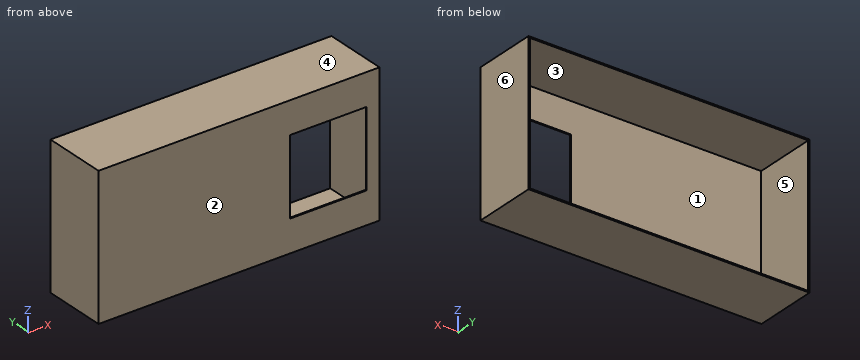
```python
from build123d import *

# Parameters (mm, degrees)
SKETCH1_W          = 2200
SKETCH1_H          = 1100
EXTRUDE1_DEPTH     = 500
SHELL1_T           = -10
SKETCH2_W          = 600
SKETCH2_H          = 600
CUT_EXTRUDE1_DEPTH = 400


with BuildPart() as part:
    # Sketch1 → Extrude1 (new body)
    with BuildSketch(Plane(origin=(0, 0, 0), x_dir=(1, 0, 0), z_dir=(0, 1, 0))):
        with Locations((-1100, 550)):
            Rectangle(SKETCH1_W, SKETCH1_H)
    extrude(amount=EXTRUDE1_DEPTH)

    # Shell1
    shell1_openings = [part.faces().sort_by_distance(p)[0] for p in [
        (-1100, 500, -550),
    ]]
    offset(amount=SHELL1_T, openings=shell1_openings, kind=Kind.INTERSECTION)

    # Sketch2 → Cut-Extrude1 (cut)
    with BuildSketch(Plane.XZ):
        with Locations((-400, -550)):
            Rectangle(SKETCH2_W, SKETCH2_H)
    extrude(amount=-CUT_EXTRUDE1_DEPTH, mode=Mode.SUBTRACT)


solid = part.part
```
Geometry check sheet. Reference: the model listing, model coordinates, mm. Face numbers are marked on the shaded views. A direction names the side the tool comes from. Coordinates: 2 decimals unless noted, no trailing zeros. Order: outer loops, then holes, each group sorted by start corner. A loop starts at its lowest first (then second) coordinate and runs counter-clockwise, first axis right, second up.
Item 1: Section check C-C (y = 61). Enter the section's corners in (x, z), plus the area to 3 significant figures.
Item 2: Scan lines: line 1 along Z through (x, y) = (-1430.5, 255); line 2 along X through (y, z) = (70.5, -101.5); line 3 along Y through (x, z) = (-1245, -1017). Record each from-to range of solid material in increasing order.
Item 3: Section check A-A (x = -139.5). Enter the section's corners in (y, z), plus the area to 3 significant figures.
Item 4: Tool access check on the marked faces 1 and 2. Record the directions out of +Z, -Z, +X, -X, +Y, -Y that give a thin tool (end or side, any length) a straight path to the whole face; none if there is none.
Item 5: Section check D-D (z = -992.5). Enter the section's corners in (x, y), plus the area to 3 significant figures.
Item 6: Mould release check, pull along Z, two halves, no side actions. Record for the marked faces 3, 4, 5 and 6: released by +Z, released by -Z, zero draft, split by the parting line, or undercut.
Item 7: Section check B-B (z = -816.5). Enter the section's corners in (x, y), plus the area to 3 significant figures.
Check sheet entries:
1. outline: (-2200, -1100) - (0, -1100) - (0, 0) - (-2200, 0) - close; hole (-2190, -1090) - (-10, -1090) - (-10, -10) - (-2190, -10) - close
1. area: 65,600 mm2
2. line 1: z = -1100 to -1090, -10 to 0
2. line 2: x = -2200 to -2190, -10 to 0
2. line 3: y = 0 to 10
3. outline: (0, -1100) - (500, -1100) - (500, -1090) - (10, -1090) - (10, -850) - (0, -850) - close; (0, -250) - (10, -250) - (10, -10) - (500, -10) - (500, 0) - (0, 0) - close
3. area: 14,800 mm2
4. face 1: +Y
4. face 2: +Z, -Z, +X, -X, -Y
5. outline: (-2200, 0) - (0, 0) - (0, 500) - (-10, 500) - (-10, 10) - (-2190, 10) - (-2190, 500) - (-2200, 500) - close
5. area: 31,800 mm2
6. face 3: undercut
6. face 4: released by +Z
6. face 5: undercut
6. face 6: zero draft
7. outline: (-2200, 0) - (-700, 0) - (-700, 10) - (-2190, 10) - (-2190, 500) - (-2200, 500) - close; (-100, 0) - (0, 0) - (0, 500) - (-10, 500) - (-10, 10) - (-100, 10) - close
7. area: 25,800 mm2
